Work out the finished part from the listing and answer in its coordinate system (mm). Round coordinates to 2 decimals unless told otherwise and drop trailing zeros. Write each loop counter-clockwise with the first axis right and the second up, starting at its lowest first coordinate (ties: lowest second). Pieces come first, ordered by that corner, then holes. Notation, with made-up numbers: (62.25, 8) -> (107.25, 8) arc R13 ccw to (107.25, 15) -> close; hole circle Ø5 at (-4.75, 10.5). An arc over 180 degrees is marked (long way). One line per question, with ' | ' between items. Start each with the question number.
```python
from build123d import *

# Parameters (mm, degrees)
SKETCH_1_R         = 3
EXTRUDE_1_DEPTH    = 10
CHAMFER_1_SIZE     = 0.1
HOLE_WIZARD_M3_1_D = 2.5


with BuildPart() as part:
    # 草图1 → 凸台-拉伸1 (new, symmetric)
    with BuildSketch(Plane.XY):
        Circle(SKETCH_1_R)
    extrude(amount=EXTRUDE_1_DEPTH, both=True)

    # 倒角1
    chamfer_1_edges = [part.edges().sort_by_distance(p)[0] for p in [
        (-3, 0, -10),
        (-3, 0, 10),
    ]]
    chamfer(chamfer_1_edges, length=CHAMFER_1_SIZE)

    # M3 螺纹孔1 (through all)
    with Locations(Plane.XY.offset(10)):
        with Locations((0, 0)):
            Hole(HOLE_WIZARD_M3_1_D / 2)


solid = part.part
```
(1) The mould has two halves that part along X. Classify faces 1 (the flat face through (1, -1, 10)), 2 (the cylindrical face through (-3, 0, 0)), 3 (the cylindrical face through (0.27, -1.22, -0.14)): +X half, -X half, draft (parallel to the pull), parting line (faces both ways), or undercut.
(2) Consider L1, parallel to Y at x = 0, z = -4; L2, parallel to X at y = 0.95, z = 0.25; L3, parallel to X at y = 1.3, z = -2. Determine where each line is inside the solid, lowest interval first.
(3) Given pin 1 Ø1 at (x, z) = (1.5, 1) entering from -Y; pin 2 Ø1 at (x, z) = (-1, -2.5) entering from +Y, each flat-ended and moving along its own axis, determine where each tip first touches the part or whether it passes through.
(4) A cutting plane is placed at A-A, the plane x = 0. Determine the outline of the cut face in (y, z).
(5) A cutting plane is placed at C-C, the plane z = -4.25. Determine the outline of the cut face in (x, y).
Returned:
1) face 1: draft | face 2: parting line | face 3: undercut
2) L1: -3 to -1.25, 1.25 to 3 | L2: -2.85 to -0.81, 0.81 to 2.85 | L3: -2.7 to 2.7
3) pin 1: y = -2.83 | pin 2: y = 2.96
4) outline: (-3, -9.9) -> (-2.9, -10) -> (-1.25, -10) -> (-1.25, 10) -> (-2.9, 10) -> (-3, 9.9) -> close; (1.25, -10) -> (2.9, -10) -> (3, -9.9) -> (3, 9.9) -> (2.9, 10) -> (1.25, 10) -> close
5) outline: circle Ø6 at (0, 0); hole circle Ø2.5 at (0, 0)
